Part model, mm, in its own coordinate system. A direction names the side the tool comes from. Round coordinates to 2 decimals unless told otherwise and drop trailing zeros. Loops run counter-clockwise (first coordinate to the right, second up) from the corner with the lowest first, then second, coordinate; pieces in that order, holes last. Notation, with made-up numbers: (55, 53) - (69, 53) arc R17 cw to (69, 84) - close; hole circle Ø9 at (15, 12.5). An arc over 180 degrees is marked (long way). Write each question's results on one line, items separated by ' | '. Start each with the question number.
(1) Mould opens along X. For faces 1 (the face through (75.49, -3.94, -75.72)), 2 (the face through (60.95, -3.94, -61.28)), 3 (the face through (-80, -316, 1)) say: released by +X, released by -X, zero draft, split by the parting line, or undercut.
(2) Tool access for faces 4 (the face through (61, -8, -58)), 5 (the face through (-73.9, -157.87, 30.64)), 6 (the face through (58, -8, 64)): list every direction of +Z, -Z, +X, -X, +Y, -Y with a clear straight run to the whole face (end or side of a thin tool).
(3) Cut at A-A, the plane z = -5. List the corners of the cut face in (x, y).
(4) Drill centre lines: L1, parallel to Z at x = 0, y = -70; L2, parallel to Y at x = -60, z = 68.5; L3, parallel to Z at x = 65, y = -316. Where is each one in solid material? Low to high.
(5) Cut at C-C, the plane z = -25. List the corners of the cut face in (x, y), then the cut area to 3 significant figures.
(6) Cut at B-B, the plane y = -245. List the corners of the cut face in (x, z).
(7) Flat gauge pins, fed straight in: P1, Ø2, axis at y = -140, z = 37, coming from the -X side; P2, Ø6, axis at x = -57.5, y = -36, coming from the +Z side; P3, Ø12, axis at y = -138.5, z = -57, coming from the -X side. Where does each tip first touch, or does it go through?
from build123d import *

# Parameters (mm, degrees)
F1_R     = 5.5
F1_R_2   = 75
F2_DEPTH = 8
F3_DEPTH = 320
F4_START = 312
F4_DEPTH = 8


with BuildPart() as f2:
    # F1 (on Front) → F2 (new body)
    with BuildSketch(Plane.XZ):
        with BuildLine():
            Line((0, -80), (65, -80))
            ThreePointArc((65, -80), (75.6066017178, -75.6066017178), (80, -65))
            Line((80, -65), (80, 0))
            ThreePointArc((80, 0), (56.5685424949, -56.5685424949), (0, -80))
        make_face()
        with Locations((65, -65)):
            Circle(F1_R, mode=Mode.SUBTRACT)
        with BuildLine():
            Line((-65, -80), (0, -80))
            ThreePointArc((0, -80), (-56.5685424251, -56.5685425648), (-80, -1.976e-07))
            Line((-80, -1.976e-07), (-80, -65))
            ThreePointArc((-80, -65), (-75.6066017178, -75.6066017178), (-65, -80))
        make_face()
        with Locations((-65, -65)):
            Circle(F1_R, mode=Mode.SUBTRACT)
        with BuildLine():
            ThreePointArc((-80, -1.976e-07), (-56.5685424251, -56.5685425648), (0, -80))
            ThreePointArc((0, -80), (56.5685424949, -56.5685424949), (80, 0))
            ThreePointArc((80, 0), (56.5685424949, 56.5685424949), (0, 80))
            ThreePointArc((0, 80), (-56.5685425648, 56.5685424251), (-80, -1.976e-07))
        make_face()
        Circle(F1_R_2, mode=Mode.SUBTRACT)
        with BuildLine():
            Line((-80, 65), (-80, -1.976e-07))
            ThreePointArc((-80, -1.976e-07), (-56.5685425648, 56.5685424251), (0, 80))
            Line((0, 80), (-65, 80))
            ThreePointArc((-65, 80), (-75.6066017178, 75.6066017178), (-80, 65))
        make_face()
        with Locations((-65, 65)):
            Circle(F1_R, mode=Mode.SUBTRACT)
        with BuildLine():
            ThreePointArc((0, 80), (56.5685424949, 56.5685424949), (80, 0))
            Line((80, 0), (80, 65))
            ThreePointArc((80, 65), (75.6066017178, 75.6066017178), (65, 80))
            Line((65, 80), (0, 80))
        make_face()
        with Locations((65, 65)):
            Circle(F1_R, mode=Mode.SUBTRACT)
    extrude(amount=F2_DEPTH)

    # F1 (on Front) → F3 (join, through all)
    with BuildSketch(Plane.XZ):
        with BuildLine():
            ThreePointArc((-80, -1.976e-07), (-56.5685424251, -56.5685425648), (0, -80))
            ThreePointArc((0, -80), (56.5685424949, -56.5685424949), (80, 0))
            ThreePointArc((80, 0), (56.5685424949, 56.5685424949), (0, 80))
            ThreePointArc((0, 80), (-56.5685425648, 56.5685424251), (-80, -1.976e-07))
        make_face()
        Circle(F1_R_2, mode=Mode.SUBTRACT)
    extrude(amount=F3_DEPTH)

    # F1 (on Front) → F4 (join)
    with BuildSketch(Plane.XZ.offset(F4_START)):
        with BuildLine():
            Line((0, -80), (65, -80))
            ThreePointArc((65, -80), (75.6066017178, -75.6066017178), (80, -65))
            Line((80, -65), (80, 0))
            ThreePointArc((80, 0), (56.5685424949, -56.5685424949), (0, -80))
        make_face()
        with Locations((65, -65)):
            Circle(F1_R, mode=Mode.SUBTRACT)
        with BuildLine():
            Line((-65, -80), (0, -80))
            ThreePointArc((0, -80), (-56.5685424251, -56.5685425648), (-80, -1.976e-07))
            Line((-80, -1.976e-07), (-80, -65))
            ThreePointArc((-80, -65), (-75.6066017178, -75.6066017178), (-65, -80))
        make_face()
        with Locations((-65, -65)):
            Circle(F1_R, mode=Mode.SUBTRACT)
        with BuildLine():
            ThreePointArc((0, 80), (56.5685424949, 56.5685424949), (80, 0))
            Line((80, 0), (80, 65))
            ThreePointArc((80, 65), (75.6066017178, 75.6066017178), (65, 80))
            Line((65, 80), (0, 80))
        make_face()
        with Locations((65, 65)):
            Circle(F1_R, mode=Mode.SUBTRACT)
        with BuildLine():
            Line((-80, 65), (-80, -1.976e-07))
            ThreePointArc((-80, -1.976e-07), (-56.5685425648, 56.5685424251), (0, 80))
            Line((0, 80), (-65, 80))
            ThreePointArc((-65, 80), (-75.6066017178, 75.6066017178), (-80, 65))
        make_face()
        with Locations((-65, 65)):
            Circle(F1_R, mode=Mode.SUBTRACT)
    extrude(amount=F4_DEPTH)


solid = f2.part
A:
1) face 1: released by +X | face 2: undercut | face 3: released by -X
2) face 4: -Z, +X | face 5: none | face 6: +Z, +X
3) outline: (-80, -320) - (-74.83, -320) - (-74.83, 0) - (-80, 0) - (-80, -8) - (-79.84, -8) - (-79.84, -312) - (-80, -312) - close; (74.83, -320) - (80, -320) - (80, -312) - (79.84, -312) - (79.84, -8) - (80, -8) - (80, 0) - (74.83, 0) - close
4) L1: -80 to -75, 75 to 80 | L2: -320 to -312, -8 to 0 | L3: -80 to -70.5, -59.5 to -37.42, 37.42 to 59.5, 70.5 to 80
5) outline: (-80, -320) - (-70.71, -320) - (-70.71, 0) - (-80, 0) - (-80, -8) - (-75.99, -8) - (-75.99, -312) - (-80, -312) - close; (70.71, -320) - (80, -320) - (80, -312) - (75.99, -312) - (75.99, -8) - (80, -8) - (80, 0) - (70.71, 0) - close | area: 3,510 mm2
6) outline: circle Ø160 at (0, 0); hole circle Ø150 at (0, 0)
7) P1: x = -71.44 | P2: z = 58.56 | P3: x = -61.64
